The drawing under review shows one solid part. Ordinate dimensions are in mm from its lowest x, y, z. A direction names the side the tool comes from. Coordinates: 2 decimals unless noted, no trailing zeros. Order: outer loops, then holes, each group sorted by start corner. A loop starts at its lowest first (then second) coordinate and runs counter-clockwise, first axis right, second up. Notation, with made-up numbers: (76, -20.5) -> (87, -20.5) arc R11 ccw to (87, -7.5) -> close; hole circle Ø11 at (-16, 76.25). An arc over 180 degrees is marked (long way). Put each result on its own line as item: value.
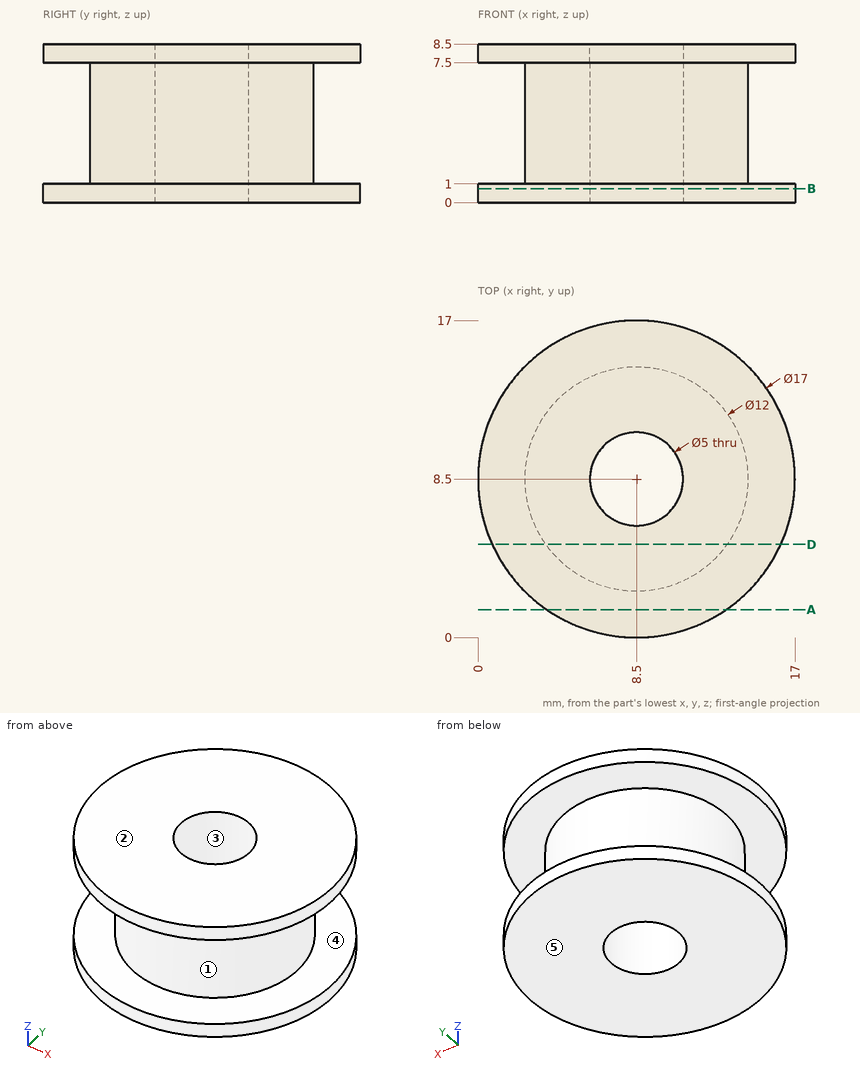
Item 1: For pin 1 Ø1.5 at (x, z) = (11, 7) entering from -Y; pin 2 Ø1.5 at (y, z) = (8, 4) entering from +X, all flat-tipped, find the tip position at first contact; note any pin that passes through.
Answers below:
pin 1: y = 0.22
pin 2: x = 14.5
Item 2: For line 1 (Z direction, x = 13.75, y = 5.5); line 2 (Y direction, x = 8.5, z = 4); line 3 (X direction, y = 8.75, z = 3.25), list the stretches that pass through material, from the lowest coordinate up. Write a range as from..to.
Answers below:
line 1: 0..1, 7.5..8.5
line 2: 2.5..6, 11..14.5
line 3: 2.51..6.01, 10.99..14.49
Item 3: Mouldability with a two-part tool opening along Y and no side actions: class the marked faces 1, 2 and 3 as +Y half, -Y half, draft (parallel to the pull), parting line (faces both ways), or undercut.
Answers below:
face 1: parting line
face 2: draft
face 3: undercut
Item 4: Consider section D-D on y = 5. Write out the cut boundary in (x, z).
Answers below:
outline: (0.75, 0) -> (16.25, 0) -> (16.25, 1) -> (13.37, 1) -> (13.37, 7.5) -> (16.25, 7.5) -> (16.25, 8.5) -> (0.75, 8.5) -> (0.75, 7.5) -> (3.63, 7.5) -> (3.63, 1) -> (0.75, 1) -> close
Item 5: For the marked faces 4 and 5, list the 3-axis set-ups (+Z, -Z, +X, -X, +Y, -Y) from which the entire face can be reached by the end or side of a thin tool; tool diameter is ignored.
Answers below:
face 4: none
face 5: -Z, +X, -X, +Y, -Y
Item 6: Consider section A-A on y = 1.5. Write out the cut boundary in (x, z).
Answers below:
outline: (3.68, 0) -> (13.32, 0) -> (13.32, 1) -> (3.68, 1) -> close; (3.68, 7.5) -> (13.32, 7.5) -> (13.32, 8.5) -> (3.68, 8.5) -> close
Item 7: Consider section B-B on z = 0.75. Write out the cut boundary in (x, y).
Answers below:
outline: circle Ø17 at (8.5, 8.5); hole circle Ø5 at (8.5, 8.5)
